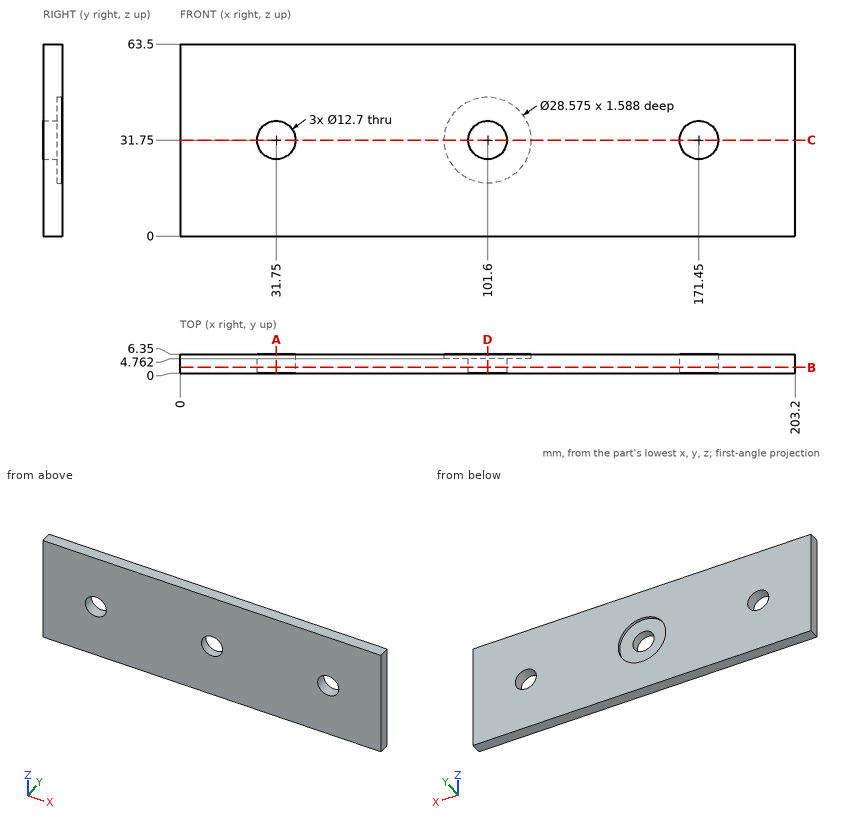
Answer from the drawing. Dimensions are ordinates in mm from the lowest x, y and z of the part. Round coordinates to 2 decimals unless told otherwise and drop trailing zeros. Write each loop counter-clockwise with the first axis right and the second up, starting at its lowest first coordinate (ties: lowest second). Pieces come first, ordered by that corner, then holes. Notation, with made-up numbers: M -28.75,77.25 L 19.25,77.25 A5 cw 19.25,84.25 Z; hole C -14.75,1 d10. An arc over 180 degrees is marked long. Write each question's results on one line, items separated by ' | '. Start each with the question number.
Item 1: Find section A-A on x = 31.75. Write down the section's boundary in (y, z).
Item 2: Find section D-D on x = 101.6. Write down the section's boundary in (y, z).
Item 3: Straight lines are drawn through the part: probe 1 along X at (y, z) = (4.5, 31.75); probe 2 along X at (y, z) = (5, 31.75); probe 3 along Z at (x, y) = (31.75, 2). For each, find the intervals that lie inside material, in ascending order.
Item 4: Find section B-B on y = 2. Write down the section's boundary in (x, z), and give its area (3 significant figures).
Item 5: Find section C-C on z = 31.75. Write down the section's boundary in (x, y), and give its area (3 significant figures).
Answer block:
1) outline: M 0,0 L 6.35,0 L 6.35,25.4 L 0,25.4 Z; M 0,38.1 L 6.35,38.1 L 6.35,63.5 L 0,63.5 Z
2) outline: M 0,0 L 6.35,0 L 6.35,17.46 L 4.76,17.46 L 4.76,25.4 L 0,25.4 Z; M 0,38.1 L 4.76,38.1 L 4.76,46.04 L 6.35,46.04 L 6.35,63.5 L 0,63.5 Z
3) probe 1: x = 0 to 25.4, 38.1 to 95.25, 107.95 to 165.1, 177.8 to 203.2 | probe 2: x = 0 to 25.4, 38.1 to 87.31, 115.89 to 165.1, 177.8 to 203.2 | probe 3: z = 0 to 25.4, 38.1 to 63.5
4) outline: M 0,0 L 203.2,0 L 203.2,63.5 L 0,63.5 Z; hole C 31.75,31.75 d12.7; hole C 101.6,31.75 d12.7; hole C 171.45,31.75 d12.7 | area: 12,500 mm²
5) outline: M 0,0 L 25.4,0 L 25.4,6.35 L 0,6.35 Z; M 38.1,0 L 95.25,0 L 95.25,4.76 L 87.31,4.76 L 87.31,6.35 L 38.1,6.35 Z; M 107.95,0 L 165.1,0 L 165.1,6.35 L 115.89,6.35 L 115.89,4.76 L 107.95,4.76 Z; M 177.8,0 L 203.2,0 L 203.2,6.35 L 177.8,6.35 Z | area: 1,020 mm²
